```python
from build123d import *

# Parameters (mm, degrees)
BOSS_EXTRUDE1_DEPTH      = 170
SKETCH7_W                = 5
SKETCH7_H                = 112.5
BOSS_EXTRUDE2_DEPTH      = 130
SKETCH9_W                = 160
SKETCH9_H                = 130
CUT_EXTRUDE2_DEPTH       = 60
SKETCH10_W               = 165
SKETCH10_H               = 3.7
CUT_EXTRUDE3_DEPTH       = 137.5
SKETCH13_W               = 160
SKETCH13_H               = 6
CUT_EXTRUDE4_DEPTH       = 5
SKETCH15_W               = 20
SKETCH15_H               = 10
BOSS_EXTRUDE3_DEPTH      = 70
SKETCH16_W               = 25
SKETCH16_H               = 12.5
CUT_EXTRUDE5_DEPTH       = 5
M6_CLEARANCE_HOLE1_D     = 7
M6_CLEARANCE_HOLE1_DEPTH = 10
SKETCH26_W               = 30
SKETCH26_H               = 9.35
CUT_EXTRUDE6_DEPTH       = 68.2
SKETCH27_W               = 30
SKETCH27_H               = 9.35
CUT_EXTRUDE8_DEPTH       = 68.2
CUT_EXTRUDE10_DEPTH      = 5
CUT_EXTRUDE11_DEPTH      = 5
SKETCH30_W               = 30
SKETCH30_H               = 9.35
CUT_EXTRUDE12_DEPTH      = 68.2
CUT_EXTRUDE14_DEPTH      = 54.5
FILLET1_R                = 2


with BuildPart() as part:
    # Sketch1 → Boss-Extrude1 (new body)
    with BuildSketch(Plane(origin=(0, 0, 0), x_dir=(0, 0, -1), z_dir=(1, 0, 0))):
        Polygon((90, 112.5), (90, 0), (85, 0), (85, 107.5), (-45, 107.5), (-45, 0), (-50, 0), (-50, 112.5), align=None)
    extrude(amount=BOSS_EXTRUDE1_DEPTH)

    # Sketch7 → Boss-Extrude2 (add)
    with BuildSketch(Plane(origin=(0, 0, 45), x_dir=(-1, 0, 0), z_dir=(0, 0, -1))):
        with Locations((-167.5, 56.25)):
            Rectangle(SKETCH7_W, SKETCH7_H)
        with Locations((-2.5, 56.25)):
            Rectangle(SKETCH7_W, SKETCH7_H)
    extrude(amount=BOSS_EXTRUDE2_DEPTH)

    # Sketch9 → Cut-Extrude2 (cut)
    with BuildSketch(Plane(origin=(0, 122.5, 0), x_dir=(1, 0, 0), z_dir=(0, 1, 0))):
        with Locations((85, 20)):
            Rectangle(SKETCH9_W, SKETCH9_H)
    extrude(amount=-CUT_EXTRUDE2_DEPTH, mode=Mode.SUBTRACT)

    # Sketch10 → Cut-Extrude3 (cut)
    with BuildSketch(Plane(origin=(80, 0, -90), x_dir=(1, 0, 0), z_dir=(0, 0, 1))):
        with Locations((5, 107.65)):
            Rectangle(SKETCH10_W, SKETCH10_H)
    extrude(amount=CUT_EXTRUDE3_DEPTH, mode=Mode.SUBTRACT)

    # Sketch13 → Cut-Extrude4 (cut)
    with BuildSketch(Plane(origin=(80, 0, -90), x_dir=(1, 0, 0), z_dir=(0, 0, 1))):
        with Locations((5, 109.5)):
            Rectangle(SKETCH13_W, SKETCH13_H)
    extrude(amount=CUT_EXTRUDE4_DEPTH, mode=Mode.SUBTRACT)

    # Sketch15 → Boss-Extrude3 (add, symmetric)
    with BuildSketch(Plane.XY.offset(-20)):
        with Locations((-10, 5)):
            Rectangle(SKETCH15_W, SKETCH15_H)
        with Locations((180, 5)):
            Rectangle(SKETCH15_W, SKETCH15_H)
    extrude(amount=BOSS_EXTRUDE3_DEPTH, both=True)

    # Sketch16 → Cut-Extrude5 (cut)
    with BuildSketch(Plane.XY.offset(50)):
        with Locations((35, 85)):
            Rectangle(SKETCH16_W, SKETCH16_H)
        with Locations((135, 85)):
            Rectangle(SKETCH16_W, SKETCH16_H)
    cut_extrude5 = extrude(amount=-CUT_EXTRUDE5_DEPTH, mode=Mode.SUBTRACT)

    # M6 Clearance Hole1
    with Locations(Plane(origin=(0, 10, 0), x_dir=(1, 0, 0), z_dir=(0, 1, 0))):
        with Locations((-10, -15), (-10, 55), (180, 55), (180, -15)):
            Hole(M6_CLEARANCE_HOLE1_D / 2, depth=M6_CLEARANCE_HOLE1_DEPTH)

    # Mirror2: Cut-Extrude5 across plane
    add(cut_extrude5.mirror(Plane.XY.offset(-20)), mode=Mode.SUBTRACT)

    # Sketch26 → Cut-Extrude6 (cut, symmetric)
    with BuildSketch(Plane.XY.offset(-20)):
        with Locations((135, 98)):
            Rectangle(SKETCH26_W, SKETCH26_H)
        with Locations((35, 98)):
            Rectangle(SKETCH26_W, SKETCH26_H)
    extrude(amount=CUT_EXTRUDE6_DEPTH, both=True, mode=Mode.SUBTRACT)

    # Sketch27 → Cut-Extrude8 (cut)
    with BuildSketch(Plane.XY.offset(-20)):
        with Locations((85, 21.8)):
            Rectangle(SKETCH27_W, SKETCH27_H)
    extrude(amount=CUT_EXTRUDE8_DEPTH, mode=Mode.SUBTRACT)

    # Sketch28 → Cut-Extrude10 (cut)
    with BuildSketch(Plane(origin=(0, 0, 50), x_dir=(-1, 0, 0), z_dir=(0, 0, -1))):
        with BuildLine():
            Line((-72.5, 0), (-72.5, 13))
            ThreePointArc((-72.5, 13), (-73.085786438, 14.414213562), (-74.5, 15))
            Line((-74.5, 15), (-95.5, 15))
            ThreePointArc((-95.5, 15), (-96.914213562, 14.414213562), (-97.5, 13))
            Line((-97.5, 13), (-97.5, 0))
            Line((-97.5, 0), (-72.5, 0))
        make_face()
    extrude(amount=CUT_EXTRUDE10_DEPTH, mode=Mode.SUBTRACT)

    # Sketch29 → Cut-Extrude11 (cut)
    with BuildSketch(Plane.XY.offset(-90)):
        with BuildLine():
            Line((95.5, 52.5), (74.5, 52.5))
            ThreePointArc((74.5, 52.5), (73.085786438, 53.085786438), (72.5, 54.5))
            Line((72.5, 54.5), (72.5, 68))
            ThreePointArc((72.5, 68), (73.085786438, 69.414213562), (74.5, 70))
            Line((74.5, 70), (95.5, 70))
            ThreePointArc((95.5, 70), (96.914213562, 69.414213562), (97.5, 68))
            Line((97.5, 68), (97.5, 54.5))
            ThreePointArc((97.5, 54.5), (96.914213562, 53.085786438), (95.5, 52.5))
        make_face()
    extrude(amount=CUT_EXTRUDE11_DEPTH, mode=Mode.SUBTRACT)

    # Sketch30 → Cut-Extrude12 (cut)
    with BuildSketch(Plane.XY.offset(-20)):
        with Locations((85, 76.8)):
            Rectangle(SKETCH30_W, SKETCH30_H)
    extrude(amount=-CUT_EXTRUDE12_DEPTH, mode=Mode.SUBTRACT)

    # Sketch31 → Cut-Extrude14 (cut)
    with BuildSketch(Plane(origin=(0, 0, 0), x_dir=(1, 0, 0), z_dir=(0, 1, 0))):
        Polygon((97.5, 86.25), (100.5, 86.25), (100.5, 88.75), (97.5, 88.75), (97.5, 90), (72.5, 90), (72.5, 88.75), (69.5, 88.75), (69.5, 86.25), (72.5, 86.25), (72.5, 85), (97.5, 85), align=None)
    extrude(amount=CUT_EXTRUDE14_DEPTH, mode=Mode.SUBTRACT)

    # Fillet1
    fillet1_edges = [part.edges().sort_by_distance(p)[0] for p in [
        (0, 61.25, 50),
        (0, 112.5, -20),
        (0, 61.25, -90),
        (-10, 10, -90),
        (0, 10, -20),
        (-20, 5, -90),
        (-20, 10, -20),
        (-10, 10, 50),
        (-20, 5, 50),
        (190, 5, -90),
        (180, 10, -90),
        (190, 10, -20),
        (170, 10, -20),
        (190, 5, 50),
        (180, 10, 50),
        (85, 112.5, 50),
        (170, 61.25, -90),
        (170, 112.5, -20),
        (170, 61.25, 50),
    ]]
    fillet(fillet1_edges, radius=FILLET1_R)


solid = part.part
```
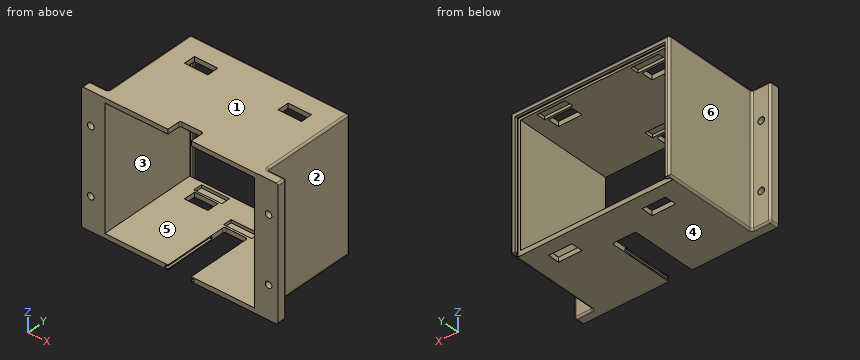
Source: CAD feature listing. Evaluate the final solid. Frame: model axes, mm. Face numbers are marked on the shaded views. A direction names the side the tool comes from. Coordinates: 2 decimals unless noted, no trailing zeros. Write each loop counter-clockwise with the first axis right and the second up, starting at its lowest first coordinate (ties: lowest second). Pieces come first, ordered by that corner, then holes. Notation, with made-up numbers: (51.25, 78) -> (74.25, 78) arc R11 cw to (74.25, 90) -> close; hole circle Ø2 at (48, 45). An arc over 180 degrees is marked (long way). Return JSON: item names as keys, results as strings. Group by question number.
1) Section query A-A, the plane x = 114. Return loops of the section in (y, z), plus the area to 3 significant figures.
2) Section query D-D, the plane x = -10. Return loops of the section in (y, z), plus the area to 3 significant figures.
3) Set-up query: the marked faces 1, 2 and 3. Return all of +Z, -Z, +X, -X, +Y, -Y with unobstructed straight access to the full face (end or side cutting, diameter ignored); none if empty.
4) Mould query, pull axis Z, two halves, no side actions, for the marked faces 4, 5 and 6. Classes: +Z half, -Z half, draft (parallel to the pull), parting line (faces both ways), or undercut.
5) Section query B-B, the plane y = 89. Return loops of the section in (x, z), plus the area to 3 significant figures.
6) Section query C-C, the plane z = 15. State how many separate pieces and enclosed holes the cut face has, plus the area to 3 significant figures.
7) Contact query for flat-ended pins moving along their axis: P1, Ø4, axis at y = 94.5, z = -25, coming from the -X side; P2, Ø5.5, axis at y = 18, z = -88, coming from the +X side; P3, Ø3.5, axis at x = 85, z = 46, coming from the -Y side. Output: stop coordinate, or through.
8) Ray query, line 1 along Z through (x, y) = (180, 6.25); line 2 along X through (y, z) = (8, 15); line 3 along X through (y, z) = (33, 16). Return the intervals inside material, ascending.
From the geometry:
{
 "1": {"outline": "(0, -90) -> (105.8, -90) -> (105.8, -85) -> (0, -85) -> close; (0, 45) -> (105.8, 45) -> (105.8, 47.5) -> (109.5, 47.5) -> (109.5, 45) -> (112.5, 45) -> (112.5, 48) arc R2 ccw to (110.5, 50) -> (0, 50) -> close", "area": "1,080 mm²"},
 "2": {"outline": "(0, -90) -> (8, -90) arc R2 ccw to (10, -88) -> (10, -58.5) -> (0, -58.5) -> close; (0, -51.5) -> (10, -51.5) -> (10, 11.5) -> (0, 11.5) -> close; (0, 18.5) -> (10, 18.5) -> (10, 48) arc R2 ccw to (8, 50) -> (0, 50) -> close", "area": "1,260 mm²"},
 "3": {"face 1": "+Z, +X, -X, +Y, -Y", "face 2": "+Z, -Z, +X, +Y", "face 3": "+Y, -Y"},
 "4": {"face 4": "-Z half", "face 5": "undercut", "face 6": "draft"},
 "5": {"outline": "(0, -88) arc R2 ccw to (2, -90) -> (22.5, -90) -> (22.5, -85) -> (5, -85) -> (5, 45) -> (22.5, 45) -> (22.5, 50) -> (2, 50) arc R2 ccw to (0, 48) -> close; (47.5, -90) -> (122.5, -90) -> (122.5, -85) -> (47.5, -85) -> close; (47.5, 45) -> (122.5, 45) -> (122.5, 50) -> (47.5, 50) -> close; (147.5, -90) -> (168, -90) arc R2 ccw to (170, -88) -> (170, 48) arc R2 ccw to (168, 50) -> (147.5, 50) -> (147.5, 45) -> (165, 45) -> (165, -85) -> (147.5, -85) -> close", "area": "2,500 mm²"},
 "6": {"separate pieces": "4", "enclosed holes": "0", "area": "1,360 mm²"},
 "7": {"P1": "x = 0", "P2": "x = 170", "P3": "y = 15"},
 "8": {"line 1": "-90 to -58.5, -51.5 to 11.5, 18.5 to 50", "line 2": "-20 to -13.5, -6.5 to 5, 165 to 176.5, 183.5 to 190", "line 3": "0 to 5, 165 to 170"}
}
